Verification items for the finished model (mm, model axes). A direction names the side the tool comes from. Round coordinates to 2 decimals unless told otherwise and drop trailing zeros. Write each loop counter-clockwise with the first axis right and the second up, starting at its lowest first coordinate (ties: lowest second). Pieces come first, ordered by that corner, then holes. Notation, with made-up numbers: (-9.75, 75) -> (7.25, 75) arc R22 cw to (7.25, 90) -> close; hole circle Ø9 at (21, 62.25). An arc over 180 degrees is marked (long way). Answer as a JSON object with one key per item and string values. Group by question number.
(1) Scan lines: L1, parallel to Z at x = 0, y = -11 (3 decimals); L2, parallel to Z at x = -16.5, y = 9.5; L3, parallel to Y at x = 24, z = 1.5. Record each from-to range of solid material in increasing order. Write a range as from..to.
(2) Gauge pin test, flat ends, axial feed: pin 1 Ø10 at (x, z) = (-5.5, 11) entering from +Y; pin 2 Ø6 at (x, z) = (0, -5.7) entering from +Y; pin 3 Ø1 at (x, y) = (8.5, -31) entering from +Z; pin 4 Ø1.5 at (x, y) = (14.5, -23.5) entering from +Z. Record the tip position at first contact, or that the pin passes through.
(3) Sectioned sample at C-C on y = 11. Record the cut outline in (x, z).
(4) Sectioned sample at A-A on x = 0. Record the cut outline in (y, z) (3 decimals), and give its area (4 significant figures).
(5) Sectioned sample at B-B on z = -5.7. Record the cut outline in (x, y) (3 decimals).
(6) Sectioned sample at D-D on z = -14. Record the cut outline in (x, y).
(7) Draft check along Z on faces 3 (the face through (17, 15, -19)), 4 (the face through (17.71, 7.6, -21.81)), 5 (the face through (-18.47, 7.6, 16.9)), 6 (the face through (12.9, -27.7, 16)). Enter one of: released by +Z, released by -Z, zero draft, split by the parting line, or undercut.
(8) Set-up check for faces 1 (the face through (-17, 15, 15)), 2 (the face through (15.93, 7.6, 16.9)): record each of +Z, -Z, +X, -X, +Y, -Y from which the full face is reachable in a straight line by a thin tool's end or side.
```python
from build123d import *

# Parameters (mm, degrees)
F0_W     = 60
F0_H     = 54
F1_DEPTH = 40
F2_R     = 2.5
F3_DEPTH = 15
F3_TAPER = 1
F4_R     = 3.375
F5_DEPTH = 40
F8_W     = 83.198
F8_H     = 59.4474617392
F9_DEPTH = 25


with BuildPart() as f1:
    # F0 (on Front) → F1 (new body)
    with BuildSketch(Plane.XZ):
        Rectangle(F0_W, F0_H)
    extrude(amount=F1_DEPTH)

    # F2 (on face) → F3 (join)
    with BuildSketch(Plane(origin=(0, 0, 0), x_dir=(-1, 0, 0), z_dir=(0, 1, 0))):
        with Locations((-17.2, 14.9)):
            Circle(F2_R)
        with Locations((17.2, 14.9)):
            Circle(F2_R)
        with Locations((17.2, -19.5)):
            Circle(F2_R)
        with Locations((-17.2, -19.5)):
            Circle(F2_R)
    extrude(amount=F3_DEPTH, taper=F3_TAPER)

    # F4 (on face) → F5 (cut, through all)
    with BuildSketch(Plane.XZ.offset(40)):
        with Locations((0, -5.7)):
            Circle(F4_R)
    extrude(amount=-F5_DEPTH, mode=Mode.SUBTRACT)

    # F8 (on 3pt) → F9 (cut)
    with BuildSketch(Plane(origin=(10.9913305692, -16.4869958538, 24.4251790426), x_dir=(0.9369493608, 0.1955162685, -0.2896537311), z_dir=(0.3494651559, -0.5241977339, 0.7765892354))):
        with Locations((-3.7034322848, -10.5544058606)):
            Rectangle(F8_W, F8_H)
    extrude(amount=F9_DEPTH, mode=Mode.SUBTRACT)


solid = f1.part
```
Computed values:
{
 "1": {"L1": "-27..-9.075, -2.325..27", "L2": "-21.73..-17.27, 12.67..17.13", "L3": "-40..0"},
 "2": {"pin 1": "y = 0", "pin 2": "through", "pin 3": "z = 16.16", "pin 4": "z = 18.72"},
 "3": {"outline": "circle Ø4.62 at (-17.2, -19.5); circle Ø4.62 at (-17.2, 14.9); circle Ø4.62 at (17.2, -19.5); circle Ø4.62 at (17.2, 14.9)"},
 "4": {"outline": "(-40, -27) -> (0, -27) -> (0, -9.075) -> (-40, -9.075) -> close; (-40, -2.325) -> (0, -2.325) -> (0, 27) -> (-20, 27) -> (-40, 13.5) -> close", "area": "1,755 mm2"},
 "5": {"outline": "(-30, -40) -> (-3.375, -40) -> (-3.375, 0) -> (-30, 0) -> close; (3.375, -40) -> (30, -40) -> (30, 0) -> (3.375, 0) -> close"},
 "6": {"outline": "(-30, -40) -> (30, -40) -> (30, 0) -> (-30, 0) -> close"},
 "7": {"face 3": "zero draft", "face 4": "undercut", "face 5": "undercut", "face 6": "released by +Z"},
 "8": {"face 1": "+Z, -Z, +X, -X, +Y", "face 2": "+Y"}
}
